from build123d import *

# Parameters (mm, degrees)
BOSS_EXTRU_1_DEPTH = 5


with BuildPart() as part:
    # Esquisse1 → Boss.-Extru.1 (new body)
    with BuildSketch(Plane(origin=(0, 0, 0), x_dir=(1, 0, 0), z_dir=(0, 1, 0))):
        with BuildLine():
            ThreePointArc((-68.670306383, 42.279177512), (-89.686678349, 4.155942482), (-85.987250464, -39.218971617))
            Line((-85.987250464, -39.218971617), (-82.83716136, -36.273074377))
            ThreePointArc((-82.83716136, -36.273074377), (-84.826823628, -30.09859374), (-86.244619049, -23.768283856))
            ThreePointArc((-86.244619049, -23.768283856), (-69.212709026, 0.560999754), (-44.883425416, -16.470910269))
            ThreePointArc((-44.883425416, -16.470910269), (-43.446659296, -1.166342783), (-34.389436177, 11.253834034))
            ThreePointArc((-34.389436177, 11.253834034), (-63.898789522, 14.600185058), (-60.552438498, 44.109538403))
            Line((-60.552438498, 44.109538403), (-62.574572693, 46.648950451))
            ThreePointArc((-62.574572693, 46.648950451), (-65.787242564, 44.693960448), (-68.670306383, 42.279177512))
        make_face()
    extrude(amount=BOSS_EXTRU_1_DEPTH)


solid = part.part
The listing builds one solid part. Answer for the finished solid, in the listing's coordinates (mm). A direction names the side the tool comes from. Give positions to 0.01 mm unless a question says otherwise; leave off trailing zeros. Write each loop counter-clockwise with the first axis right and the second up, starting at its lowest first coordinate (ties: lowest second). Pieces come first, ordered by that corner, then holes. Notation, with made-up numbers: (10.5, 26.5) - (14.5, 26.5) arc R35 cw to (14.5, 60.5) - close; hole circle Ø2 at (46, -0.75). An arc over 180 degrees is marked (long way). One line per question, with ' | ' between items. Start each with the question number.
1. Section A-A, the plane z = 1 is taken. Determine the outline of the cut face in (x, y), then the cut area to 3 significant figures.
2. Section B-B, the plane x = -66 is taken. Determine the outline of the cut face in (y, z), then the cut area to 3 significant figures.
3. For faces 5 (the face through (-71, 5, -7)), 6 (the face through (-84.8, 2.5, 30.2)), determine the directions among +Z, -Z, +X, -X, +Y, -Y from which every point of the face is accessible in a straight line to the end or side of a thin tool.
4. Determine the mould class of faces 1 (the face through (-84.434, 2.465, 37.767)), 2 (the face through (-69.667, 2.465, -0.476)), 3 (the face through (-89.556, 2.465, -4.76)), 4 (the face through (-61.55, 2.46, -45.36)) for opening direction Z: +Z half, -Z half, draft (parallel to the pull), parting line (faces both ways), or undercut.
5. Straight lines are drawn through the part: line 1 (X direction, y = 1.55, z = 1.5); line 2 (Z direction, x = -61.5, y = 4.8); line 3 (X direction, y = 0.3, z = 7). For each, find the intervals that lie inside material, in ascending order.
6. Section C-C, the plane y = 3.95 is taken. Determine the outline of the cut face in (x, z).
7. Section D-D, the plane x = -39.5 is taken. Determine the outline of the cut face in (y, z).
8. Given P1, Ø2, axis at x = -84.5, z = 25, coming from the -Y side; P2, Ø1, axis at y = 2, z = -35, coming from the +X side; P3, Ø2, axis at x = -49, y = 2.5, coming from the +Z side; P4, Ø3, axis at y = 2.5, z = -20.5, coming from the +X side, each flat-ended and moving along its own axis, determine where each tip first touches the part or whether it passes through.
Result:
1) outline: (-90.6, 0) - (-74.25, 0) - (-74.25, 5) - (-90.6, 5) - close; (-56.88, 0) - (-43.38, 0) - (-43.38, 5) - (-56.88, 5) - close | area: 149 mm2
2) outline: (0, -44.54) - (5, -44.54) - (5, -37.56) - (0, -37.56) - close; (0, -17.8) - (5, -17.8) - (5, -0.88) - (0, -0.88) - close | area: 119 mm2
3) face 5: +Z, -Z, +X, -X, +Y | face 6: +X, +Y, -Y
4) face 1: +Z half | face 2: undercut | face 3: parting line | face 4: -Z half
5) line 1: x = -90.66 to -75.28, -55.85 to -43.57 | line 2: z = -45.3 to -43.31, -12.06 to -0.48 | line 3: x = -91.19 to -81.96, -49.17 to -44.98
6) outline: (-86.24, 23.77) arc R71 cw to (-82.84, 36.27) - (-85.99, 39.22) arc R75 ccw to (-68.67, -42.28) arc R25 ccw to (-62.57, -46.65) - (-60.55, -44.11) arc R21 cw to (-34.39, -11.25) arc R29 cw to (-44.88, 16.47) arc R21 cw to start
7) outline: (0, -8.25) - (5, -8.25) - (5, -6) - (0, -6) - close
8) P1: passes through | P2: stops at x = -66.96 | P3: stops at z = 8.61 | P4: stops at x = -66.59
